```python
from build123d import *

# Parameters (mm, degrees)
BOSS_EXTRUDE1_DEPTH = 10


with BuildPart() as part:
    # Sketch1 → Boss-Extrude1 (new body)
    with BuildSketch(Plane.XY):
        with BuildLine():
            Line((1.447213595, 99.276393202), (97.88854382, 51.05572809))
            ThreePointArc((97.88854382, 51.05572809), (100.06315057, 50.267510105), (102.360679775, 50))
            Line((102.360679775, 50), (755, 50))
            ThreePointArc((755, 50), (758.535533906, 48.535533906), (760, 45))
            Line((760, 45), (760, -45.000000001))
            ThreePointArc((760, -45.000000001), (758.535533906, -48.535533907), (755, -50.000000001))
            Line((755, -50.000000001), (102.360679777, -50.000000001))
            ThreePointArc((102.360679777, -50.000000001), (100.06315057, -50.267510107), (97.888543818, -51.055728093))
            Line((97.888543818, -51.055728093), (80.530859307, -59.734570358))
            ThreePointArc((80.530859307, -59.734570358), (79.995557001, -59.964284692), (79.437170731, -60.130182272))
            ThreePointArc((79.437170731, -60.130182272), (29.605594549, -91.672663918), (10.00115127, -147.294421683))
            ThreePointArc((10.00115127, -147.294421683), (9.977672992, -147.753763522), (9.912084694, -148.209004479))
            Line((9.912084694, -148.209004479), (1.982173893, -189.643070819))
            ThreePointArc((1.982173893, -189.643070819), (0.90559103, -190.450629734), (0, -189.455096236))
            Line((0, -189.455096236), (0, 98.381966011))
            ThreePointArc((0, 98.381966011), (0.474268888, 99.23261682), (1.447213595, 99.276393202))
        make_face()
    extrude(amount=BOSS_EXTRUDE1_DEPTH)


solid = part.part
```
Geometry: final body of the model. Coordinates: model frame, mm. Coordinates: 2 decimals unless noted, no trailing zeros. Order: outer loops, then holes, each group sorted by start corner. A loop starts at its lowest first (then second) coordinate and runs counter-clockwise, first axis right, second up. Notation, with made-up numbers: (83, -12.5) -> (115, -12.5) arc R6 ccw to (115, -5.5) -> close; hole circle Ø3 at (78.25, 74). An arc over 180 degrees is marked (long way). Answer in a Markdown table with one row per item.
Item 1: Section C-C on y = -155. Output: boundary loops of the cut face in (x, z), plus the area to 3 significant figures.
Return value:
| item | result |
|---|---|
| outline | (0, 0) -> (8.61, 0) -> (8.61, 10) -> (0, 10) -> close |
| area | 86.1 mm² |
Item 2: Ray query, L1, parallel to Y at x = 347.5, z = 7; L2, parallel to X at y = -73, z = 8; L3, parallel to X at y = 63.5, z = 7. Return the intervals inside material, ascending.
Return value:
| item | result |
|---|---|
| L1 | y = -50 to 50 |
| L2 | x = 0 to 49.88 |
| L3 | x = 0 to 73 |
Item 3: Section B-B on x = 325. Output: boundary loops of the cut face in (y, z).
Return value:
| item | result |
|---|---|
| outline | (-50, 0) -> (50, 0) -> (50, 10) -> (-50, 10) -> close |
Item 4: Section A-A on z = 7.75. Output: boundary loops of the cut face in (x, y).
Return value:
| item | result |
|---|---|
| outline | (0, -189.46) arc R1 ccw to (1.98, -189.64) -> (9.91, -148.21) arc R5 ccw to (10, -147.29) arc R90 cw to (79.44, -60.13) arc R5 ccw to (80.53, -59.73) -> (97.89, -51.06) arc R10 cw to (102.36, -50) -> (755, -50) arc R5 ccw to (760, -45) -> (760, 45) arc R5 ccw to (755, 50) -> (102.36, 50) arc R10 cw to (97.89, 51.06) -> (1.45, 99.28) arc R1 ccw to (0, 98.38) -> close |
Item 5: Contact query for flat-ended pins moving along their axis: P1, Ø6, axis at y = 59.5, z = 6.5, coming from the +X side; P2, Ø4, axis at x = 149.5, z = 6.5, coming from the +Y side. Output: stop coordinate, or through.
Return value:
| item | result |
|---|---|
| P1 | stops at x = 87 |
| P2 | stops at y = 50 |
